Geometry check sheet. Reference: the model listing, model coordinates, mm. Face numbers are marked on the shaded views. A direction names the side the tool comes from. Coordinates: 2 decimals unless noted, no trailing zeros. Write each loop counter-clockwise with the first axis right and the second up, starting at its lowest first coordinate (ties: lowest second). Pieces come first, ordered by that corner, then holes. Notation, with made-up numbers: (15.25, -8) - (35.25, -8) arc R20 ccw to (35.25, 15) - close; hole circle Ø2 at (89.5, 61.5). An arc over 180 degrees is marked (long way). Answer as a JSON object with one key per item and string values. Group by question number.
from build123d import *

# Parameters (mm, degrees)
SKETCH1_R             = 1.55
BOSS_EXTRUDE1_DEPTH   = 7.9
CUT_EXTRUDE2_DEPTH    = 60.130449009
M3X0_5_TAPPED_HOLE1_D = 2.5
SKETCH7_W             = 8
SKETCH7_H             = 0.5
CUT_EXTRUDE3_DEPTH    = 60.130449009
SKETCH8_R             = 2.1
CUT_EXTRUDE4_DEPTH    = 56.645395137
CUT_EXTRUDE5_DEPTH    = 3
CUT_EXTRUDE6_DEPTH    = 1
FILLET4_R             = 0.5
FILLET5_R             = 2


with BuildPart() as part:
    # Sketch1 → Boss-Extrude1 (new body)
    with BuildSketch(Plane(origin=(0, 0, 0), x_dir=(0, 0, -1), z_dir=(1, 0, 0))):
        with BuildLine():
            Line((0, 0), (0, 16))
            Line((0, 16), (-19.367478425, 51.438690431))
            ThreePointArc((-19.367478425, 51.438690431), (-23.205351274, 52.747203725), (-24.84125158, 49.037041298))
            Line((-24.84125158, 49.037041298), (-15, 20))
            Line((-15, 20), (-15, 0))
            Line((-15, 0), (0, 0))
        make_face()
        with Locations((-22, 50)):
            Circle(SKETCH1_R, mode=Mode.SUBTRACT)
    extrude(amount=BOSS_EXTRUDE1_DEPTH)

    # Sketch3 → Cut-Extrude2 (cut, through all)
    with BuildSketch(Plane(origin=(0, 0, 0), x_dir=(-1, 0, 0), z_dir=(0, 0, -1))):
        Polygon((-7.9, 0), (-4.9, 0), (-2.9, 4), (-7.9, 4), align=None)
    extrude(amount=-CUT_EXTRUDE2_DEPTH, mode=Mode.SUBTRACT)

    # M3x0.5 Tapped Hole1 (through all)
    with Locations(Plane(origin=(7.9, 7, 3), x_dir=(0, 0, 1), z_dir=(1, 0, 0))):
        with Locations((0, 0)):
            Hole(M3X0_5_TAPPED_HOLE1_D / 2)

    # Sketch7 → Cut-Extrude3 (cut, through all)
    with BuildSketch(Plane(origin=(0, 0, 0), x_dir=(-1, 0, 0), z_dir=(0, 0, -1))):
        with Locations((-4, 0.25)):
            Rectangle(SKETCH7_W, SKETCH7_H)
    extrude(amount=-CUT_EXTRUDE3_DEPTH, mode=Mode.SUBTRACT)

    # Sketch8 → Cut-Extrude4 (cut, through all)
    with BuildSketch(Plane.XY.offset(15)):
        with Locations((3.9, 12)):
            Circle(SKETCH8_R)
    extrude(amount=-CUT_EXTRUDE4_DEPTH, mode=Mode.SUBTRACT)

    # Sketch9 → Cut-Extrude5 (cut)
    with BuildSketch(Plane(origin=(0, 0, 0), x_dir=(-1, 0, 0), z_dir=(0, 0, -1))):
        Polygon((-4.65, 0.5), (-2.9, 4), (0, 4), (0, 0.5), align=None)
    extrude(amount=-CUT_EXTRUDE5_DEPTH, mode=Mode.SUBTRACT)

    # Sketch11 → Cut-Extrude6 (cut)
    with BuildSketch(Plane.ZY):
        with BuildLine():
            Line((0, 16), (15, 20))
            Line((15, 20), (24.84125158, 49.037041298))
            ThreePointArc((24.84125158, 49.037041298), (23.205351274, 52.747203725), (19.367478425, 51.438690431))
            Line((19.367478425, 51.438690431), (0, 16))
        make_face()
    extrude(amount=-CUT_EXTRUDE6_DEPTH, mode=Mode.SUBTRACT)

    # Fillet4
    fillet4_edges = [part.edges().sort_by_distance(p)[0] for p in [
        (1, 18, 7.5),
        (0, 18, 7.5),
    ]]
    fillet(fillet4_edges, radius=FILLET4_R - 0.0001)  # a hair under: the kernel refuses the full size

    # Fillet5
    fillet5_edges = [part.edges().sort_by_distance(p)[0] for p in [
        (5.4, 4, 15),
        (3.95, 4, 0),
    ]]
    fillet(fillet5_edges, radius=FILLET5_R)


solid = part.part
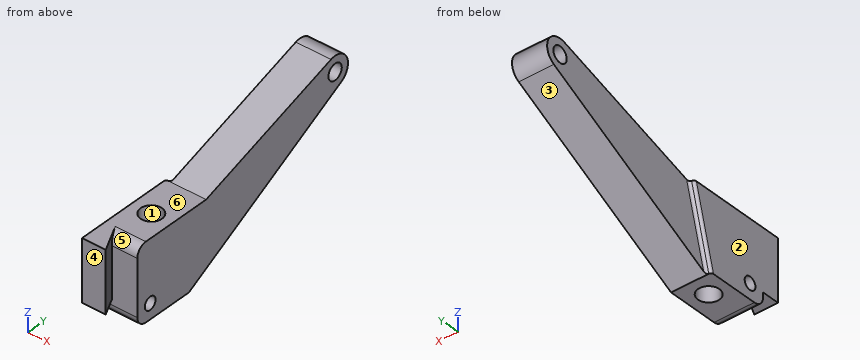
(1) Section check C-C (z = 22.75). Record the cut outline in (x, y).
(2) Draft check along Y on the marked faces 1, 2 and 3. Enter one of: +Y half, -Y half, draft (parallel to the pull), parting line (faces both ways), or undercut.
(3) Material ranges on L1, parallel to Z at x = 5.5, y = 7; L2, parallel to Y at x = 3, z = 2.75; L3, parallel to Y at x = 3, z = 3.25, recorded low to high. Write a range as [from, to].
(4) Section check A-A (x = 3.9). Record the cut outline in (y, z).
(5) Gauge pin test, flat ends, axial feed: pin 1 (1 mm diameter, centred on x = 7, z = 20, fed in from +Y); pin 2 (2.5 mm diameter, centred on x = 4.5, y = 6.5, fed in from +Z); pin 3 (5 mm diameter, centred on y = 25, z = 7, fed in from -X); pin 4 (3 mm diameter, centred on y = 7, z = 3, fed in from -X). Record the tip position at first contact, or that the pin passes through.
(6) Set-up check for the marked faces 4, 5 and 6: record each of +Z, -Z, +X, -X, +Y, -Y from which the full face is reachable in a straight line by a thin tool's end or side.
(7) Section check D-D (z = 18.5). Record the cut outline in (x, y), and give its area (3 significant figures).
(8) Section check B-B (y = 7). Record the cut outline in (x, z).
Conclusion:
{
 "1": {"outline": "(1, 42.87) - (7.9, 42.87) - (7.9, 48.64) - (1, 48.64) - close; (1, 51.36) - (7.9, 51.36) - (7.9, 52.9) - (1, 52.9) - close"},
 "2": {"face 1": "undercut", "face 2": "draft", "face 3": "+Y half"},
 "3": {"L1": "z = [0, 1.75], [4.25, 15]", "L2": "y = [4, 5.78], [8.22, 10.1], [13.9, 21.03]", "L3": "y = [0.5, 3.8], [4, 5.78], [8.22, 10.1], [13.9, 21.95]"},
 "4": {"outline": "(0.5, 3) - (2, 3) - (2, 15) - (0.5, 15) - close; (4, 2) arc R2 ccw to (6, 0) - (9.9, 0) - (9.9, 15) - (6, 15) arc R2 ccw to (4, 13) - close; (14.1, 0) - (16, 0) - (51.44, 19.37) arc R3 ccw to (49.04, 24.84) - (20, 15) - (14.1, 15) - close; hole circle Ø2.5 at (7, 3); hole circle Ø3.1 at (50, 22)"},
 "5": {"pin 1": "stops at y = 52.6", "pin 2": "stops at z = 15", "pin 3": "stops at x = 1", "pin 4": "stops at x = 0"},
 "6": {"face 4": "+Z, -Z, +X, -X, -Y", "face 5": "+Z, +X", "face 6": "+Z, +X, -X, -Y"},
 "7": {"outline": "(1, 30.33) - (7.9, 30.33) - (7.9, 49.85) - (1, 49.85) - close", "area": "135 mm^2"},
 "8": {"outline": "(0, 0) - (7.9, 0) - (7.9, 1.75) - (0, 1.75) - close; (0, 4.25) - (7.9, 4.25) - (7.9, 15) - (0, 15) - close"}
}
